from build123d import *

# Parameters (mm, degrees)
EXTRUDE_1_DEPTH = 32
EXTRUDE_2_DEPTH = 25
EXTRUDE_3_DEPTH = 15


with BuildPart() as part:
    # Sketch 1 → Extrude 1 (new body)
    with BuildSketch(Plane(origin=(0, 0, 0), x_dir=(1, 0, 0), z_dir=(0, 1, 0))):
        with BuildLine():
            ThreePointArc((15, -20), (22.360679775, -11.180339887), (25, 0))
            ThreePointArc((25, 0), (22.360679775, 11.180339887), (15, 20))
            ThreePointArc((15, 20), (-25, 0), (15, -20))
        make_face()
        with BuildLine():
            Line((-20, 0), (-20, 4))
            Line((-20, 4), (-14.456832295, 4))
            ThreePointArc((-14.456832295, 4), (15, 0), (-14.456832295, -4))
            Line((-14.456832295, -4), (-20, -4))
            Line((-20, -4), (-20, 0))
        make_face(mode=Mode.SUBTRACT)
    extrude(amount=EXTRUDE_1_DEPTH)

    # Sketch 1_3 → Extrude 2 (add)
    with BuildSketch(Plane(origin=(0, 0, 0), x_dir=(1, 0, 0), z_dir=(0, 1, 0))):
        with BuildLine():
            Line((31, 0), (25, 0))
            ThreePointArc((25, 0), (22.360679775, -11.180339887), (15, -20))
            Line((15, -20), (76, -20))
            Line((76, -20), (76, -14))
            Line((76, -14), (36.124783736, -14))
            ThreePointArc((36.124783736, -14), (31.445906532, -11.756076158), (30.266710698, -6.702702703))
            ThreePointArc((30.266710698, -6.702702703), (30.816132396, -3.371347532), (31, 0))
        make_face()
        with BuildLine():
            ThreePointArc((15, 20), (22.360679775, 11.180339887), (25, 0))
            Line((25, 0), (31, 0))
            ThreePointArc((31, 0), (30.816132396, 3.371347532), (30.266710698, 6.702702703))
            ThreePointArc((30.266710698, 6.702702703), (31.445906532, 11.756076158), (36.124783736, 14))
            Line((36.124783736, 14), (76, 14))
            Line((76, 14), (76, 20))
            Line((76, 20), (15, 20))
        make_face()
    extrude(amount=EXTRUDE_2_DEPTH)

    # Sketch 1_4 → Extrude 3 (add)
    with BuildSketch(Plane(origin=(0, 0, 0), x_dir=(1, 0, 0), z_dir=(0, 1, 0))):
        with BuildLine():
            ThreePointArc((30.266710698, 6.702702703), (30.816132396, 3.371347532), (31, 0))
            ThreePointArc((31, 0), (30.816132396, -3.371347532), (30.266710698, -6.702702703))
            ThreePointArc((30.266710698, -6.702702703), (31.445906532, -11.756076158), (36.124783736, -14))
            Line((36.124783736, -14), (76, -14))
            Line((76, -14), (76, 0))
            Line((76, 0), (76, 14))
            Line((76, 14), (36.124783736, 14))
            ThreePointArc((36.124783736, 14), (31.445906532, 11.756076158), (30.266710698, 6.702702703))
        make_face()
        with BuildLine():
            ThreePointArc((41, 0), (46, 5), (51, 0))
            ThreePointArc((51, 0), (46, -5), (41, 0))
        make_face(mode=Mode.SUBTRACT)
        with BuildLine():
            ThreePointArc((59, 0), (64, 5), (69, 0))
            ThreePointArc((69, 0), (64, -5), (59, 0))
        make_face(mode=Mode.SUBTRACT)
    extrude(amount=EXTRUDE_3_DEPTH)


solid = part.part
Build history of the part. All positions in model axes, mm. A direction names the side the tool comes from. Give positions to 0.01 mm unless a question says otherwise; leave off trailing zeros. Write each loop counter-clockwise with the first axis right and the second up, starting at its lowest first coordinate (ties: lowest second). Pieces come first, ordered by that corner, then holes. Notation, with made-up numbers: (62.25, 57) - (111.25, 57) arc R18 ccw to (111.25, 75) - close; hole circle Ø3 at (61.5, 41). An arc over 180 degrees is marked (long way). Use one line per item in the form item = value. Start each with the question number.
1. Two-plate mould, pull along Z, no slides. Class faces 1 (the face through (-17, 16, 4)), 2 (the face through (30, 25, 0)), 3 (the face through (46, 12, -20)), 4 (the face through (56, 20, 14)): released by +Z, released by -Z, zero draft, split by the parting line, or undercut.
2. Drop flat-ended pins along their axis: pin 1 Ø7.5 at (x, y) = (46, 12) entering from -Z; pin 2 Ø3 at (x, z) = (10.5, -7) entering from -Y; pin 3 Ø22.5 at (x, z) = (61.5, -3) entering from +Y; pin 4 Ø8 at (y, z) = (21, -6.5) entering from -X. Give the stop position or say it passes through.
3. Band-saw the part on C-C on z = -12. Write the cut outline in (x, y), plus the area to 3 significant figures.
4. Probe line 1 (Z direction, x = 64, y = 7); line 2 (Z direction, x = 38, y = 17.5); line 3 (Y direction, x = 38.5, z = 11). List the from-to ranges inside material, lowest first. Write a range as [from, to].
5. Band-saw the part on D-D on x = 0. Write the cut outline in (y, z).
6. 3-axis set-ups, long thin cutter, end or side, ignore diameter. For faces 5 (the face through (-20, 16, 0)), 6 (the face through (45, 12, 20)), 7 (the face through (31.4, 19.9, -11.7)): which of +Z, -Z, +X, -X, +Y, -Y reach the whole face in a straight line?
7. Band-saw the part on B-B on y = 3. Write the cut outline in (x, z).
8. Band-saw the part on A-A on x = 46. Write the cut outline in (y, z), plus the area to 3 significant figures.
Conclusion:
q1.face_1 = undercut
q1.face_2 = zero draft
q1.face_3 = released by -Z
q1.face_4 = undercut
q2.pin_1 = -20
q2.pin_2 = through
q2.pin_3 = 25
q2.pin_4 = -24.87
q3.outline = (-21.93, 0) - (-9, 0) - (-9, 32) - (-21.93, 32) - close; (9, 0) - (76, 0) - (76, 15) - (31.65, 15) - (31.65, 25) - (21.93, 25) - (21.93, 32) - (9, 32) - close
q3.area = 1,740 mm²
q4.line_1 = [-20, -5], [5, 20]
q4.line_2 = [-20, -14], [14, 20]
q4.line_3 = [0, 15]
q5.outline = (0, -25) - (32, -25) - (32, -15) - (0, -15) - close; (0, 15) - (32, 15) - (32, 25) - (0, 25) - close
q6.face_5 = +Y, -Y
q6.face_6 = +Z, +X, +Y, -Y
q6.face_7 = +X, +Y
q7.outline = (15, -20) - (76, -20) - (76, 20) - (15, 20) arc R25 ccw (long way) to start; hole (-20, -4) - (-14.46, -4) arc R15 ccw (long way) to (-14.46, 4) - (-20, 4) - close; hole circle Ø10 at (46, 0); hole circle Ø10 at (64, 0)
q8.outline = (0, -20) - (25, -20) - (25, -14) - (15, -14) - (15, -5) - (0, -5) - close; (0, 5) - (15, 5) - (15, 14) - (25, 14) - (25, 20) - (0, 20) - close
q8.area = 570 mm²
